Geometry: final body of the model. Coordinates: model frame, mm. Face numbers are marked on the shaded views. A direction names the side the tool comes from. Round coordinates to 2 decimals unless told otherwise and drop trailing zeros. Write each loop counter-clockwise with the first axis right and the second up, starting at its lowest first coordinate (ties: lowest second). Pieces come first, ordered by that corner, then holes.
from build123d import *

# Parameters (mm, degrees)
F0_W     = 200
F0_H     = 200
F1_DEPTH = 200
F3_DEPTH = 150
F4_DEPTH = 25


with BuildPart() as f1:
    # F0 (on Front) → F1 (new body)
    with BuildSketch(Plane.XZ):
        with Locations((100, 100)):
            Rectangle(F0_W, F0_H)
        with BuildLine():
            ThreePointArc((100, 145), (131.8198051534, 131.8198051534), (145, 100))
            ThreePointArc((145, 100), (68.1801948466, 68.1801948466), (100, 145))
        make_face(mode=Mode.SUBTRACT)
    extrude(amount=F1_DEPTH)

    # F2 (on Top) → F3 (cut)
    with BuildSketch(Plane.XY):
        with BuildLine():
            ThreePointArc((100, -175), (153.033008589, -153.033008589), (175, -100))
            ThreePointArc((175, -100), (46.966991411, -46.966991411), (100, -175))
        make_face()
    extrude(amount=F3_DEPTH, mode=Mode.SUBTRACT)

    # F0 (on Front) → F4 (join)
    with BuildSketch(Plane.XZ):
        with BuildLine():
            ThreePointArc((100, 145), (68.1801948466, 68.1801948466), (145, 100))
            ThreePointArc((145, 100), (131.8198051534, 131.8198051534), (100, 145))
        make_face()
    extrude(amount=F4_DEPTH)


solid = f1.part
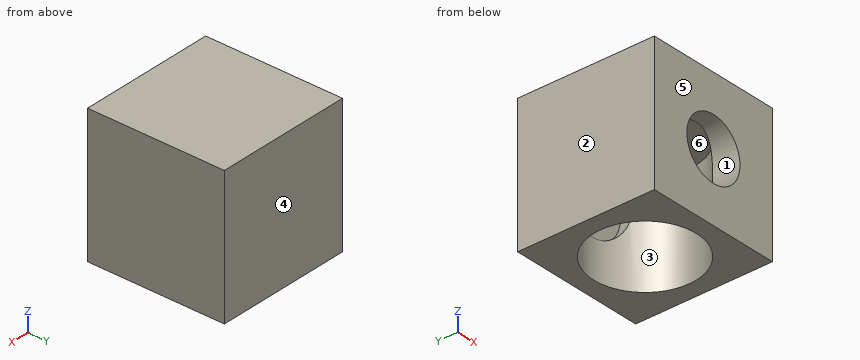
1) Draft query along Y for the marked faces 4, 5 and 6. Return one class per face: pulls with the +Y half, pulls with the -Y half, needs draft (parallel to the pull), parting line crosses it, or undercut.
2) Reachability of the marked faces 1, 2 and 3 from +Z, -Z, +X, -X, +Y, -Y: full face, straight path, thin tool, end or side. Return the list, or none.
3) Section C-C on z = 100. Output: boundary loops of the cut face in (x, y).
4) Line query: probe 1 along X at (y, z) = (-182, 100); probe 2 along Y at (x, z) = (100, 45.5). Output: solid intervals per line, ascending.
5) First-contact query: P1, Ø3, axis at y = -130.5, z = 32.5, coming from the -X side; P2, Ø6, axis at x = 133, y = -127.5, coming from the -Z side. Flat tips, straight axial feed; report the tip coordinate or a pass-through.
6) Section D-D on y = -100. Output: boundary loops of the cut face in (x, z), plus the area to 3 significant figures.
7) Section A-A on x = 160. Output: boundary loops of the cut face in (y, z), plus the area to 3 significant figures.
8) Section B-B on x = 67. Output: boundary loops of the cut face in (y, z), plus the area to 3 significant figures.
Filled in:
1. face 4: pulls with the +Y half
1. face 5: pulls with the -Y half
1. face 6: undercut
2. face 1: -Y
2. face 2: +Z, -Z, -X, +Y, -Y
2. face 3: -Z
3. outline: (0, -200) - (55, -200) - (55, -160) arc R75 cw to (55, -40) - (55, -25) - (145, -25) - (145, -40) arc R75 cw to (145, -160) - (145, -200) - (200, -200) - (200, 0) - (0, 0) - close
4. probe 1: x = 0 to 55, 145 to 200
4. probe 2: y = -200 to -175, -25 to 0
5. P1: stops at x = 0
5. P2: stops at z = 150
6. outline: (0, 0) - (25, 0) - (25, 150) - (175, 150) - (175, 0) - (200, 0) - (200, 200) - (0, 200) - close
6. area: 17,500 mm2
7. outline: (-200, 0) - (-145, 0) - (-145, 150) - (-55, 150) - (-55, 0) - (0, 0) - (0, 200) - (-200, 200) - close
7. area: 26,500 mm2
8. outline: (-200, 0) - (-167.35, 0) - (-167.35, 69.41) - (-200, 69.41) - close; (-200, 130.59) - (-167.35, 130.59) - (-167.35, 150) - (-32.65, 150) - (-32.65, 130.59) - (-25, 130.59) - (-25, 69.41) - (-32.65, 69.41) - (-32.65, 0) - (0, 0) - (0, 200) - (-200, 200) - close
8. area: 17,300 mm2
